from build123d import *

# Parameters (mm, degrees)
PAD003_DEPTH      = 2
PAD003_DEPTH_BACK = 2
SKETCH019_W       = 25
SKETCH019_H       = 75
PAD018_DEPTH      = 1


with BuildPart() as body003:
    # Sketch004 → Pad003 (new body, two sides)
    with BuildSketch(Plane.XY) as pad003_sk:
        Polygon((12.5, 65.625), (3.125, 9.375), (21.875, 9.375), align=None)
    extrude(amount=PAD003_DEPTH)
    extrude(pad003_sk.sketch, amount=-PAD003_DEPTH_BACK)


with BuildPart() as body017:
    # Sketch019 → Pad018 (new body)
    with BuildSketch(Plane.XY):
        with Locations((12.5, 37.5)):
            Rectangle(SKETCH019_W, SKETCH019_H)
    extrude(amount=PAD018_DEPTH)

    # Boolean002: cut Body003
    add(body003.part, mode=Mode.SUBTRACT)


solid = body017.part
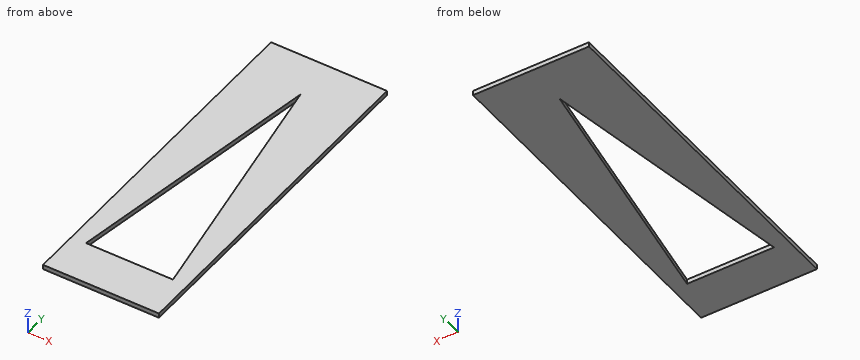
Read the model definition and answer for the solid it produces. Units are mm, in the model's axes. Round coordinates to 2 decimals unless told otherwise and drop trailing zeros. Order: outer loops, then holes, each group sorted by start corner. A loop starts at its lowest first (then second) coordinate and runs counter-clockwise, first axis right, second up.
1) The part is cut by section C-C on z = 0.75. Write down the section's boundary in (x, y) (3 decimals).
2) The part is cut by section B-B on x = 18. Write down the section's boundary in (y, z) (3 decimals), plus the area to 4 significant figures.
3) Straight lines are drawn through the part: L1, parallel to X at y = 26, z = 0.9; L2, parallel to X at y = 64.5, z = 0.55. For each, find the intervals that lie inside material, in ascending order.
4) The part is cut by section A-A on y = 17. Write down the section's boundary in (x, z).
5) A flat-ended cylindrical pin translates along its axis: pin 1 (1.5 mm diameter, centred on x = 22.5, y = 21, fed in from -Z). Find the tip coordinate at first contact, or state that the pin passes through.
Resolved:
1. outline: (0, 0) - (25, 0) - (25, 75) - (0, 75) - close; hole (3.125, 9.375) - (21.875, 9.375) - (12.5, 65.625) - close
2. outline: (0, 0) - (9.375, 0) - (9.375, 1) - (0, 1) - close; (32.625, 0) - (75, 0) - (75, 1) - (32.625, 1) - close
2. area: 51.75 mm2
3. L1: x = 0 to 5.9, 19.1 to 25
3. L2: x = 0 to 12.31, 12.69 to 25
4. outline: (0, 0) - (4.4, 0) - (4.4, 1) - (0, 1) - close; (20.6, 0) - (25, 0) - (25, 1) - (20.6, 1) - close
5. pin 1: stops at z = 0
